```python
from build123d import *

# Parameters (mm, degrees)
BOSS_EXTRUDE1_DEPTH     = 36
CUT_EXTRUDE1_DEPTH      = 51.222007128
CUT_EXTRUDE1_DEPTH_BACK = 51.222007128
CUT_EXTRUDE2_DEPTH      = 51.222007128
CUT_EXTRUDE2_DEPTH_BACK = 51.222007128


with BuildPart() as part:
    # Sketch1 → Boss-Extrude1 (new, symmetric)
    with BuildSketch(Plane.XY):
        Polygon((-24, -25.5), (-4, -25.5), (-4, -12.5), (4, -12.5), (4, -25.5), (24, -25.5), (24, -4.5), (20, -4.5), (20, 4.5), (24, 4.5), (24, 25.5), (4, 25.5), (4, 4.5), (-4, 4.5), (-4, 25.5), (-24, 25.5), (-24, 4.5), (-20, 4.5), (-20, -4.5), (-24, -4.5), align=None)
    extrude(amount=BOSS_EXTRUDE1_DEPTH, both=True)

    # Sketch2 → Cut-Extrude1 (cut, two sides: drawn at the far end of the back side and taken through both)
    with BuildSketch(Plane.XY.offset(-CUT_EXTRUDE1_DEPTH_BACK)):
        Polygon((-14, 25.5), (-4, 14.197056136), (4, 14.197056136), (14, 25.5), align=None)
    extrude(amount=CUT_EXTRUDE1_DEPTH + CUT_EXTRUDE1_DEPTH_BACK, mode=Mode.SUBTRACT)

    # Sketch3 → Cut-Extrude2 (cut, two sides: drawn at the far end of the back side and taken through both)
    with BuildSketch(Plane.XY.offset(-CUT_EXTRUDE2_DEPTH_BACK)):
        Polygon((4, -17.157724852), (11, -25.5), (-11, -25.5), (-4, -17.157724852), align=None)
    extrude(amount=CUT_EXTRUDE2_DEPTH + CUT_EXTRUDE2_DEPTH_BACK, mode=Mode.SUBTRACT)


solid = part.part
```
Could you check a few things on this model? Use its own coordinates, in mm. A direction names the side the tool comes from. Coordinates: 2 decimals unless noted, no trailing zeros. Write each loop counter-clockwise with the first axis right and the second up, starting at its lowest first coordinate (ties: lowest second). Pieces come first, ordered by that corner, then holes. Notation, with made-up numbers: (-22.75, -21.75) -> (-1.75, -21.75) arc R12 cw to (-1.75, -3.75) -> close; hole circle Ø10 at (-32, 52.5). An arc over 180 degrees is marked (long way). Return JSON: item names as keys, results as strings.
(1) Imagine slicing it at C-C, the plane x = 2. Please give me the cut outline in (y, z).
Numbers:
{"outline": "(-12.5, -36) -> (4.5, -36) -> (4.5, 36) -> (-12.5, 36) -> close"}
(2) Imagine slicing it at A-A, the plane y = 12.5. Please give me the cut outline in (x, z).
Numbers:
{"outline": "(-24, -36) -> (-4, -36) -> (-4, 36) -> (-24, 36) -> close; (4, -36) -> (24, -36) -> (24, 36) -> (4, 36) -> close"}
(3) Imagine slicing it at D-D, the plane y = 18.5. Please give me the cut outline in (x, z).
Numbers:
{"outline": "(-24, -36) -> (-7.81, -36) -> (-7.81, 36) -> (-24, 36) -> close; (7.81, -36) -> (24, -36) -> (24, 36) -> (7.81, 36) -> close"}
(4) Imagine slicing it at B-B, the plane z = 14. Please give me the cut outline in (x, y), then the cut area to 3 significant figures.
Numbers:
{"outline": "(-24, -25.5) -> (-11, -25.5) -> (-4, -17.16) -> (-4, -12.5) -> (4, -12.5) -> (4, -17.16) -> (11, -25.5) -> (24, -25.5) -> (24, -4.5) -> (20, -4.5) -> (20, 4.5) -> (24, 4.5) -> (24, 25.5) -> (14, 25.5) -> (4, 14.2) -> (4, 4.5) -> (-4, 4.5) -> (-4, 14.2) -> (-14, 25.5) -> (-24, 25.5) -> (-24, 4.5) -> (-20, 4.5) -> (-20, -4.5) -> (-24, -4.5) -> close", "area": "1,930 mm2"}
(5) I'm going to push flat-ended pins straight in: pin 1 (2 mm diameter, centred on x = 13.5, z = 24, fed in from +Y); pin 2 (6 mm diameter, centred on y = 1, z = 27.5, fed in from +X); pin 3 (9 mm diameter, centred on x = 0.5, z = 12.5, fed in from -Y). Where does each tip first touch, or does it pass through?
Numbers:
{"pin 1": "stops at y = 25.5", "pin 2": "stops at x = 20", "pin 3": "stops at y = -18.35"}
(6) We'd pull the mould along Y, two halves only. Please class faces 6 (the flat face through (7.45, -21.27, -0.5)), 7 (the flat face through (20, 0, 1)), 8 (the flat face through (-4, -15, 1)): +Y half, -Y half, draft (parallel to the pull), parting line (faces both ways), or undercut.
Numbers:
{"face 6": "-Y half", "face 7": "undercut", "face 8": "draft"}
(7) I need wall thicknesses on L1, parallel to X at y = -16, z = 32.5; L2, parallel to Y at x = 21.5, z = -12; L3, parallel to X at y = 23.5, z = -14.5. Which ranges of each line are inside material? Lowest first, please.
Numbers:
{"L1": "x = -24 to -4, 4 to 24", "L2": "y = -25.5 to -4.5, 4.5 to 25.5", "L3": "x = -24 to -12.23, 12.23 to 24"}
(8) Which directions (+Z, -Z, +X, -X, +Y, -Y) give clear straight access to the entire face, cutting with the end or side of a thin tool? Please do faces 1 (the flat face through (17, -25.5, 1)), 2 (the flat face through (22, 4.5, 1)), 3 (the flat face through (-22, 4.5, 1)), 4 (the flat face through (-7.55, -21.39, -0.5)), 5 (the flat face through (-4, 9, 1)).
Numbers:
{"face 1": "+Z, -Z, +X, -X, -Y", "face 2": "+Z, -Z, +X", "face 3": "+Z, -Z, -X", "face 4": "+Z, -Z, -Y", "face 5": "+Z, -Z, +Y"}
